Drawing for the job (mm, zero at the part's lowest x, y, z). A direction names the side the tool comes from. Round coordinates to 2 decimals unless told otherwise and drop trailing zeros. Write each loop counter-clockwise with the first axis right and the second up, starting at its lowest first coordinate (ties: lowest second). Pieces come first, ordered by that corner, then holes. Notation, with made-up numbers: (50.5, 66.5) - (96.5, 66.5) arc R21 cw to (96.5, 87.5) - close; hole circle Ø11 at (-16.75, 35.25). An arc over 180 degrees is marked (long way). One line per question, with ' | ' between items.
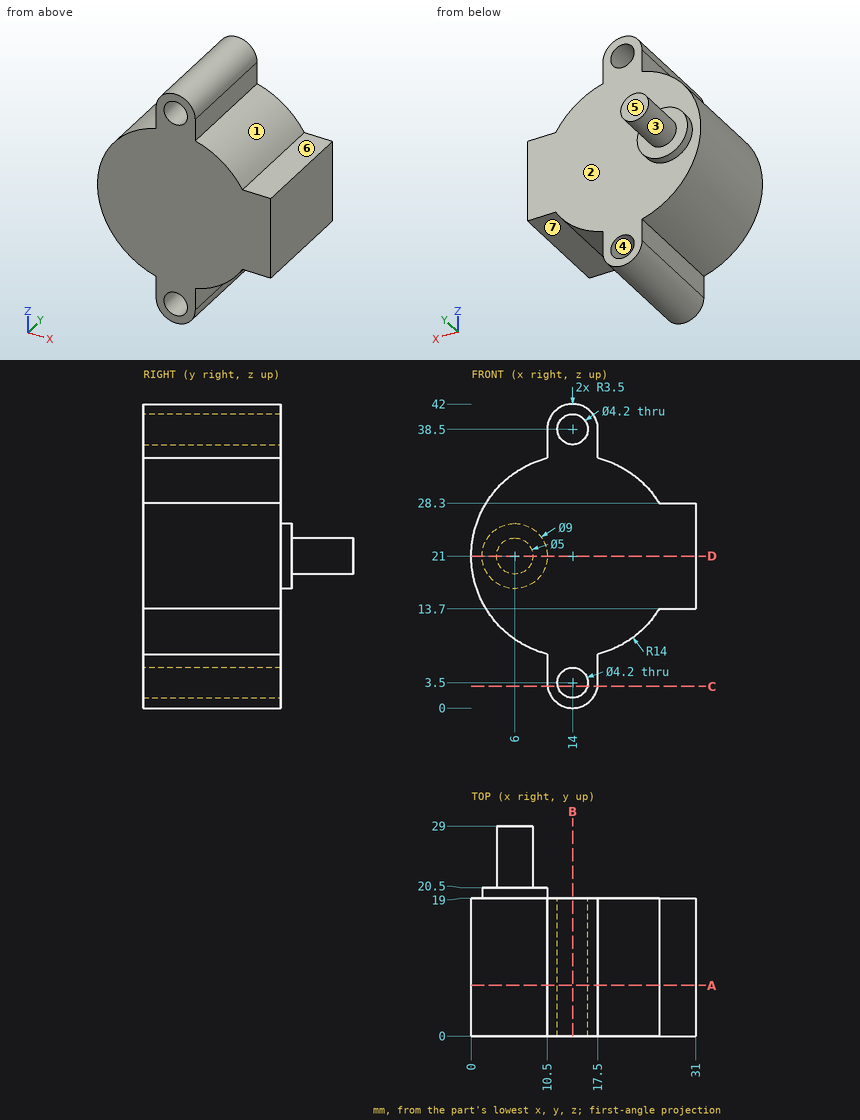
Q1. Pull direction X, two halves, no side cores. Call the marked faces 1, 2, 3 and 4: +X half, -X half, draft (parallel to the pull), parting line (faces both ways), or undercut.
Found:
face 1: +X half | face 2: draft | face 3: parting line | face 4: undercut
Q2. Which spindle directions (+Z, -Z, +X, -X, +Y, -Y) get a long thin tool onto all of the face, cutting with end or side? Do the marked faces 5, 6 and 7. Say none if no direction does.
Found:
face 5: +Z, -Z, +X, -X, +Y | face 6: +Z, +X, +Y, -Y | face 7: -Z, +X, +Y, -Y
Q3. Saw through at D-D, the plane z = 21. List the corners of the cut face in (x, y).
Found:
outline: (0, 0) - (31, 0) - (31, 19) - (10.5, 19) - (10.5, 20.5) - (8.5, 20.5) - (8.5, 29) - (3.5, 29) - (3.5, 20.5) - (1.5, 20.5) - (1.5, 19) - (0, 19) - close
Q4. Drop flat-ended pins along their axis: pin 1 (1.2 mm diameter, centred on y = 7, z = 36.5, fed in from +X); pin 2 (4 mm diameter, centred on x = 17.5, z = 33.5, fed in from -Y); pin 3 (2 mm diameter, centred on y = 6.5, z = 36.5, fed in from -X); pin 4 (4 mm diameter, centred on x = 29.5, y = 5, fed in from +Z). Give the stop position or say it passes through.
Found:
pin 1: x = 17.5 | pin 2: y = 0 | pin 3: x = 10.5 | pin 4: z = 28.3
Q5. Drill centre lines: L1, parallel to X at y = 5, z = 38.5; L2, parallel to Y at x = 11, z = 26.5; L3, parallel to X at y = 4, z = 20.5. Where is each one in solid material? Low to high. Write a range as from..to.
Found:
L1: 10.5..11.9, 16.1..17.5 | L2: 0..19 | L3: 0.01..31
Q6. Saw through at B-B, the plane x = 14. List the corners of the cut face in (y, z), then the cut area to 3 significant figures.
Found:
outline: (0, 0) - (19, 0) - (19, 1.4) - (0, 1.4) - close; (0, 5.6) - (19, 5.6) - (19, 36.4) - (0, 36.4) - close; (0, 40.6) - (19, 40.6) - (19, 42) - (0, 42) - close | area: 638 mm^2
Q7. Saw through at A-A, the plane y = 7. List the corners of the cut face in (x, z).
Found:
outline: (10.5, 3.5) arc R3.5 ccw to (17.5, 3.5) - (17.5, 7.44) arc R14 ccw to (25.95, 13.7) - (31, 13.7) - (31, 28.3) - (25.95, 28.3) arc R14 ccw to (17.5, 34.56) - (17.5, 38.5) arc R3.5 ccw to (10.5, 38.5) - (10.5, 34.56) arc R14 ccw to (10.5, 7.44) - close; hole circle Ø4.2 at (14, 3.5); hole circle Ø4.2 at (14, 38.5)
Q8. Saw through at C-C, the plane z = 3. List the corners of the cut face in (x, y), then the cut area to 3 significant figures.
Found:
outline: (10.54, 0) - (11.96, 0) - (11.96, 19) - (10.54, 19) - close; (16.04, 0) - (17.46, 0) - (17.46, 19) - (16.04, 19) - close | area: 54.1 mm^2
